```python
from build123d import *

# Parameters (mm, degrees)
F0_R     = 35.56
F1_DEPTH = 76.2
F2_W     = 25.4
F2_H     = 50.8
F3_DEPTH = 50.8
F5_R     = 7.62
F6_DEPTH = 66.04


with BuildPart() as f1:
    # F0 (on Top) → F1 (new body)
    with BuildSketch(Plane.XY):
        Circle(F0_R)
    extrude(amount=F1_DEPTH)

    # F2 (on face) → F3 (cut)
    with BuildSketch(Plane(origin=(0, 0, 0), x_dir=(1, 0, 0), z_dir=(0, 0, -1))):
        Rectangle(F2_W, F2_H)
    extrude(amount=-F3_DEPTH, mode=Mode.SUBTRACT)

    # F5 (on offset) → F6 (join)
    with BuildSketch(Plane.YZ.offset(33.02)):
        with Locations((0, 25.4)):
            Circle(F5_R)
    extrude(amount=-F6_DEPTH)


solid = f1.part
```
Can you work these out from the model? Positions are in its coordinate system, mm. A direction names the side the tool comes from. Coordinates: 2 decimals unless noted, no trailing zeros. Write each loop counter-clockwise with the first axis right and the second up, starting at its lowest first coordinate (ties: lowest second). Pieces come first, ordered by that corner, then holes. Notation, with made-up numbers: (23.25, -26.75) - (36.25, -26.75) arc R26 ccw to (36.25, 12.25) - close; hole circle Ø4 at (65.5, -23). An arc over 180 degrees is marked (long way). Return JSON: item names as keys, results as strings.
Q1. Thinking about a two-plate mould opening in Y: for faces 1 (the flat face through (15, 0, 0)), 2 (the flat face through (0, 0, 50.8)), 3 (the cylindrical face through (-7.709, -34.714, 37.567)), which applies, +Y half, -Y half, draft (parallel to the pull), parting line (faces both ways), or undercut?
Computed values:
{"face 1": "draft", "face 2": "undercut", "face 3": "parting line"}
Q2. If we section it at D-D (z = 40): Please give me the cut outline in (x, y).
Computed values:
{"outline": "circle Ø71.12 at (0, 0); hole (-12.7, -25.4) - (12.7, -25.4) - (12.7, 25.4) - (-12.7, 25.4) - close"}
Q3. If we section it at B-B (y = 0): Please give me the cut outline in (x, z), then the cut area to 3 significant figures.
Computed values:
{"outline": "(-35.56, 0) - (-12.7, 0) - (-12.7, 17.78) - (12.7, 17.78) - (12.7, 0) - (35.56, 0) - (35.56, 76.2) - (-35.56, 76.2) - close; hole (-12.7, 33.02) - (12.7, 33.02) - (12.7, 50.8) - (-12.7, 50.8) - close", "area": "4,520 mm2"}
Q4. Please list where these lines run through material, in increasing order: L1, parallel to Y at x = -1, z = 48.5; L2, parallel to X at y = 11, z = 36.5; L3, parallel to Z at x = 6.5, y = -12. Write a range as from..to.
Computed values:
{"L1": "y = -35.55..-25.4, 25.4..35.55", "L2": "x = -33.82..-12.7, 12.7..33.82", "L3": "z = 50.8..76.2"}
Q5. If we section it at C-C (z = 25.4): Please give me the cut outline in (x, y).
Computed values:
{"outline": "circle Ø71.12 at (0, 0); hole (-12.7, -25.4) - (12.7, -25.4) - (12.7, -7.62) - (-12.7, -7.62) - close; hole (-12.7, 7.62) - (12.7, 7.62) - (12.7, 25.4) - (-12.7, 25.4) - close"}
Q6. I'm going to push flat-ended pins straight in: pin 1 Ø4 at (x, z) = (0, 20.5) entering from -Y; pin 2 Ø2 at (y, z) = (-13.5, 23) entering from -X; pin 3 Ø3 at (x, z) = (8.5, 10) entering from -Y. Where does each tip first touch, or does it pass through?
Computed values:
{"pin 1": "stops at y = -35.56", "pin 2": "stops at x = -33.29", "pin 3": "stops at y = -34.86"}
Q7. If we section it at A-A (x = 0): Please give me the cut outline in (y, z).
Computed values:
{"outline": "(-35.56, 0) - (-25.4, 0) - (-25.4, 50.8) - (25.4, 50.8) - (25.4, 0) - (35.56, 0) - (35.56, 76.2) - (-35.56, 76.2) - close; circle Ø15.24 at (0, 25.4)"}
Q8. On a 3-axis mill with a long thin cutter (end or side, diameter ignored), from which of +Z, -Z, +X, -X, +Y, -Y can I reach the whole of each face in a straight line? I mean faces 4 (the cylindrical face through (0.18, -1.65, 17.96)), 5 (the flat face through (0, 0, 76.2)), 6 (the flat face through (0, -25.4, 25)). Say none if no direction works.
Computed values:
{"face 4": "none", "face 5": "+Z, +X, -X, +Y, -Y", "face 6": "-Z"}
